from build123d import *

# Parameters (mm, degrees)
SKETCH1_R                          = 16.7894
BOSS_EXTRUDE1_DEPTH                = 20
SKETCH2_W                          = 3.683
SKETCH2_H                          = 2.1082
CUT_EXTRUDE1_DEPTH                 = 21
FILLET1_R                          = 4.7625
F_3_16_0_1875_DIAMETER_HOLE1_D     = 4.7625
F_3_16_0_1875_DIAMETER_HOLE1_DEPTH = 11.543700016
F_3_16_0_1875_DIAMETER_HOLE1_TIP   = 1.430799349


with BuildPart() as part:
    # Sketch1 → Boss-Extrude1 (new body)
    with BuildSketch(Plane.XY):
        Circle(SKETCH1_R)
    extrude(amount=BOSS_EXTRUDE1_DEPTH)

    # Sketch2 → Cut-Revolve1 (revolve, cut)
    with BuildSketch(Plane(origin=(0, 0, 0), x_dir=(0, 0, -1), z_dir=(1, 0, 0))):
        with Locations((-16.1585, 15.7353)):
            Rectangle(SKETCH2_W, SKETCH2_H)
        with Locations((-3.8415, 15.7353)):
            Rectangle(SKETCH2_W, SKETCH2_H)
    revolve(axis=Axis((0, 0, 21.240749408), (0, 0, -1)), mode=Mode.SUBTRACT)

    # Sketch3 → Cut-Extrude1 (cut, through all)
    with BuildSketch(Plane.XY.offset(20)):
        with BuildLine():
            Line((-12.580888371, -2.300000032), (12.580888371, -2.300000032))
            ThreePointArc((12.580888371, -2.300000032), (0, 12.7894), (-12.580888371, -2.300000032))
        make_face()
    extrude(amount=-CUT_EXTRUDE1_DEPTH, mode=Mode.SUBTRACT)

    # Fillet1
    fillet1_edges = [part.edges().sort_by_distance(p)[0] for p in [
        (-12.580888371, -2.300000032, 10),
        (12.580888371, -2.300000032, 10),
    ]]
    fillet(fillet1_edges, radius=FILLET1_R)

    # 3/16 (0.1875) Diameter Hole1
    with Locations(Plane(origin=(0, 16.7894, 0), x_dir=(-1, 0, 0), z_dir=(0, 1, 0))):
        with Locations((0, 10)):
            Hole(F_3_16_0_1875_DIAMETER_HOLE1_D / 2, depth=F_3_16_0_1875_DIAMETER_HOLE1_DEPTH)
            with Locations((0, 0, -(F_3_16_0_1875_DIAMETER_HOLE1_DEPTH + F_3_16_0_1875_DIAMETER_HOLE1_TIP / 2))):  # 118° drill point
                Cone(0, F_3_16_0_1875_DIAMETER_HOLE1_D / 2, F_3_16_0_1875_DIAMETER_HOLE1_TIP, mode=Mode.SUBTRACT)


solid = part.part
Design review of the part built by this model. Coordinates are the model's own, in mm. A direction names the side the tool comes from. Coordinates: 2 decimals unless noted, no trailing zeros. Write each loop counter-clockwise with the first axis right and the second up, starting at its lowest first coordinate (ties: lowest second). Pieces come first, ordered by that corner, then holes. Notation, with made-up numbers: (30.5, 81) -> (61.5, 81) arc R24 ccw to (61.5, 112) -> close; hole circle Ø8 at (79.5, 56.25). An arc over 180 degrees is marked (long way). Write each question's results on one line, items separated by ' | '. Start each with the question number.
(1) Clearance check with flat-ended pins moving along their axes: P1, Ø3, axis at x = 5.5, z = 2, coming from the +Y side; P2, Ø4, axis at y = -12, z = 13, coming from the -X side; P3, Ø12, axis at y = 13.5, z = 8, coming from the +X side; P4, Ø10, axis at x = -3.5, y = 3.5, coming from the +Z side. State where each tip first meets the part, or that it passes through.
(2) Take a section at C-C on z = 7. Write out the cut boundary in (x, y) (1 decimal).
(3) The part is to be moulded in two halves that separate along Z. For faces 5 (the face through (-11.452, -0.392, 9.86)), 6 (the face through (0, -3, 0)), 7 (the face through (-15, 0, 14.317)), say which applies: pulls with the +Z half, pulls with the -Z half, needs draft (parallel to the pull), parting line crosses it, or undercut.
(4) Take a section at B-B on y = 9. Write out the cut boundary in (x, z), and give its area (3 significant figures).
(5) For line 1 along Z through (x, y) = (0, 15); line 2 along Z through (x, y) = (-9, -13); line 3 along Y through (x, z) = (-4, 1), list the stretches that pass through material, from the lowest coordinate up. Write a range as from..to.
(6) Take a section at A-A on x = 0. Write out the cut boundary in (y, z), and give its area (3 significant figures).
(7) Take a section at D-D on x = -4.5. Write out the cut boundary in (y, z).
(8) Tool access review of faces 1 (the face through (11.452, -0.392, 9.86)), 2 (the face through (2.2, 14.65, 9.09)), 3 (the face through (-15, 0, 18)), 4 (the face through (0, -3, 20)): name each direction out of +Z, -Z, +X, -X, +Y, -Y from which nothing blocks a thin tool from reaching the whole face with its end or side.
Results found:
1) P1: stops at y = 16.31 | P2: stops at x = -13.49 | P3: stops at x = 15.02 | P4: passes through
2) outline: circle Ø33.6 at (0, 0); hole (-12.2, 3.9) arc R4.8 ccw to (-7.6, -2.3) -> (7.6, -2.3) arc R4.8 ccw to (12.2, 3.9) arc R12.8 ccw to start
3) face 5: needs draft | face 6: pulls with the -Z half | face 7: undercut
4) outline: (-14.17, 0) -> (-9.09, 0) -> (-9.09, 20) -> (-14.17, 20) -> (-14.17, 18) -> (-11.6, 18) -> (-11.6, 14.32) -> (-14.17, 14.32) -> (-14.17, 5.68) -> (-11.6, 5.68) -> (-11.6, 2) -> (-14.17, 2) -> close; (9.09, 0) -> (14.17, 0) -> (14.17, 2) -> (11.6, 2) -> (11.6, 5.68) -> (14.17, 5.68) -> (14.17, 14.32) -> (11.6, 14.32) -> (11.6, 18) -> (14.17, 18) -> (14.17, 20) -> (9.09, 20) -> close | area: 166 mm2
5) line 1: z = 0..2, 5.68..7.62, 12.38..14.32, 18..20 | line 2: z = 0..2, 5.68..14.32, 18..20 | line 3: y = -16.31..-2.3, 12.15..16.31
6) outline: (-16.79, 0) -> (-2.3, 0) -> (-2.3, 20) -> (-16.79, 20) -> (-16.79, 18) -> (-14.68, 18) -> (-14.68, 14.32) -> (-16.79, 14.32) -> (-16.79, 5.68) -> (-14.68, 5.68) -> (-14.68, 2) -> (-16.79, 2) -> close; (12.79, 0) -> (16.79, 0) -> (16.79, 2) -> (14.68, 2) -> (14.68, 5.68) -> (16.79, 5.68) -> (16.79, 7.62) -> (12.79, 7.62) -> close; (12.79, 12.38) -> (16.79, 12.38) -> (16.79, 14.32) -> (14.68, 14.32) -> (14.68, 18) -> (16.79, 18) -> (16.79, 20) -> (12.79, 20) -> close | area: 320 mm2
7) outline: (-16.18, 0) -> (-2.3, 0) -> (-2.3, 20) -> (-16.18, 20) -> (-16.18, 18) -> (-13.97, 18) -> (-13.97, 14.32) -> (-16.18, 14.32) -> (-16.18, 5.68) -> (-13.97, 5.68) -> (-13.97, 2) -> (-16.18, 2) -> close; (11.97, 0) -> (16.18, 0) -> (16.18, 2) -> (13.97, 2) -> (13.97, 5.68) -> (16.18, 5.68) -> (16.18, 14.32) -> (13.97, 14.32) -> (13.97, 18) -> (16.18, 18) -> (16.18, 20) -> (11.97, 20) -> close
8) face 1: +Z, -Z | face 2: +Y | face 3: none | face 4: +Z, +X, -X, +Y, -Y
